The model under review builds one solid part; all positions refer to its coordinate system, in mm. A direction names the side the tool comes from. Coordinates: 2 decimals unless noted, no trailing zeros. Order: outer loops, then holes, each group sorted by start corner. A loop starts at its lowest first (then second) coordinate and runs counter-clockwise, first axis right, second up. Notation, with made-up numbers: (-36, 14.25) - (-4, 14.25) arc R23 ccw to (-4, 36.25) - close; hole circle Ø2 at (89, 51). An arc over 180 degrees is marked (long way). Answer in a Markdown table with one row per item.
```python
from build123d import *

# Parameters (mm, degrees)
CYLINDER009_R     = 1.5
CYLINDER009_DEPTH = 10
CYLINDER008_R     = 1.5
CYLINDER008_DEPTH = 10
CYLINDER001_R     = 3.5
CYLINDER001_DEPTH = 20
PAD_DEPTH         = 2
CYLINDER_R        = 15
CYLINDER_DEPTH    = 4.9


with BuildPart() as cilindro009:
    # Cylinder009 → Cylinder009 (new body)
    with BuildSketch(Plane(origin=(-3, 14, 24), x_dir=(1, 0, 0), z_dir=(0, 0, 1))):
        Circle(CYLINDER009_R)
    extrude(amount=CYLINDER009_DEPTH)


with BuildPart() as cilindro008:
    # Cylinder008 → Cylinder008 (new body)
    with BuildSketch(Plane(origin=(-3, -3, 24), x_dir=(1, 0, 0), z_dir=(0, 0, 1))):
        Circle(CYLINDER008_R)
    extrude(amount=CYLINDER008_DEPTH)


with BuildPart() as cilindro001:
    # Cylinder001 → Cylinder001 (new body)
    with BuildSketch(Plane(origin=(6, 6, 22), x_dir=(1, 0, 0), z_dir=(0, 0, 1))):
        Circle(CYLINDER001_R)
    extrude(amount=CYLINDER001_DEPTH)


with BuildPart() as pad:
    # Sketch → Pad (new body)
    with BuildSketch(Plane(origin=(6, 6, 31.6), x_dir=(-1, 0, 0), z_dir=(0, 0, -1))):
        with BuildLine():
            ThreePointArc((14.086174, -1.998143), (16, 0), (14.086174, 1.998143))
            Line((2.44949, 2.5), (14.086174, 1.998143))
            Line((2.44949, 2.5), (2.44949, -2.5))
            Line((2.44949, -2.5), (14.086174, -1.998143))
        make_face()
    extrude(amount=PAD_DEPTH)


with BuildPart() as base:
    # Cylinder → Cylinder (new body)
    with BuildSketch(Plane(origin=(0, 6, 26.7), x_dir=(1, 0, 0), z_dir=(0, 0, 1))):
        Circle(CYLINDER_R)
    extrude(amount=CYLINDER_DEPTH)

    # Cut: cut Pad
    add(pad.part, mode=Mode.SUBTRACT)

    # Cut001: cut Cilindro001
    add(cilindro001.part, mode=Mode.SUBTRACT)

    # Cut009: cut Cilindro008
    add(cilindro008.part, mode=Mode.SUBTRACT)

    # Cut010: cut Cilindro009
    add(cilindro009.part, mode=Mode.SUBTRACT)


solid = base.part
```
Item 1: Tool access review of faces 4 (the face through (-10, 6, 31)), 5 (the face through (-1.614, 13.425, 29.116)): name each direction out of +Z, -Z, +X, -X, +Y, -Y from which nothing blocks a thin tool from reaching the whole face with its end or side.
Check values:
| item | result |
|---|---|
| face 4 | +Z |
| face 5 | +Z, -Z |
Item 2: We need section A-A, the plane y = 6. Write out the cut boundary in (x, z).
Check values:
| item | result |
|---|---|
| outline | (-15, 26.7) - (2.5, 26.7) - (2.5, 29.6) - (-10, 29.6) - (-10, 31.6) - (-15, 31.6) - close; (9.5, 26.7) - (15, 26.7) - (15, 31.6) - (9.5, 31.6) - close |
Item 3: Clearance check with flat-ended pins moving along their axes: pin 1 Ø2 at (x, z) = (-11.5, 27.5) entering from +Y; pin 2 Ø1 at (x, z) = (-10.5, 28.5) entering from +Y; pin 3 Ø1.5 at (x, z) = (-1.5, 28.5) entering from -Y. State where each tip first meets the part, or that it passes through.
Check values:
| item | result |
|---|---|
| pin 1 | y = 16.71 |
| pin 2 | y = 17.18 |
| pin 3 | y = -8.98 |
Item 4: Mouldability with a two-part tool opening along X and no side actions: class faces 1 (the face through (9.233, 4.659, 29.116)), 2 (the face through (-1.953, 20.872, 29.116)), 3 (the face through (0, 3, 31.6)) as +X half, -X half, draft (parallel to the pull), parting line (faces both ways), or undercut.
Check values:
| item | result |
|---|---|
| face 1 | undercut |
| face 2 | parting line |
| face 3 | draft |
Item 5: We need section B-B, the plane x = -3. Write out the cut boundary in (y, z), then the cut area to 3 significant figures.
Check values:
| item | result |
|---|---|
| outline | (-8.7, 26.7) - (-4.5, 26.7) - (-4.5, 31.6) - (-8.7, 31.6) - close; (-1.5, 26.7) - (12.5, 26.7) - (12.5, 31.6) - (8.22, 31.6) - (8.22, 29.6) - (3.78, 29.6) - (3.78, 31.6) - (-1.5, 31.6) - close; (15.5, 26.7) - (20.7, 26.7) - (20.7, 31.6) - (15.5, 31.6) - close |
| area | 106 mm^2 |
Item 6: To check wall thickness, follow line 1 (Y direction, x = -3, z = 27.85); line 2 (Y direction, x = 2, z = 31); line 3 (Z direction, x = -2.5, y = 8). State the ranges of each line that lie inside material, in increasing order. Write a range as from..to.
Check values:
| item | result |
|---|---|
| line 1 | -8.7..-4.5, -1.5..12.5, 15.5..20.7 |
| line 2 | -8.87..3.57, 8.43..20.87 |
| line 3 | 26.7..29.6 |
Item 7: We need section C-C, the plane z = 30.55. Write out the cut boundary in (x, y).
Check values:
| item | result |
|---|---|
| outline | circle Ø30 at (0, 6); hole (-8.09, 4) - (3.55, 3.5) arc R3.5 ccw (long way) to (3.55, 8.5) - (-8.09, 8) arc R2 ccw to start; hole circle Ø3 at (-3, -3); hole circle Ø3 at (-3, 14) |
Item 8: We need section D-D, the plane x = 6. Write out the cut boundary in (y, z).
Check values:
| item | result |
|---|---|
| outline | (-7.75, 26.7) - (2.5, 26.7) - (2.5, 31.6) - (-7.75, 31.6) - close; (9.5, 26.7) - (19.75, 26.7) - (19.75, 31.6) - (9.5, 31.6) - close |
